Answer from the drawing. Dimensions are ordinates in mm from the lowest x, y and z of the part. Coordinates: 2 decimals unless noted, no trailing zeros. Loops run counter-clockwise (first coordinate to the right, second up) from the corner with the lowest first, then second, coordinate; pieces in that order, holes last. Notation, with made-up numbers: M 71,28.25 L 78,28.25 A16 cw 78,58.25 Z; hole C 70.5,30 d11. An arc over 180 degrees is marked long. Put each result on its own line as item: value.
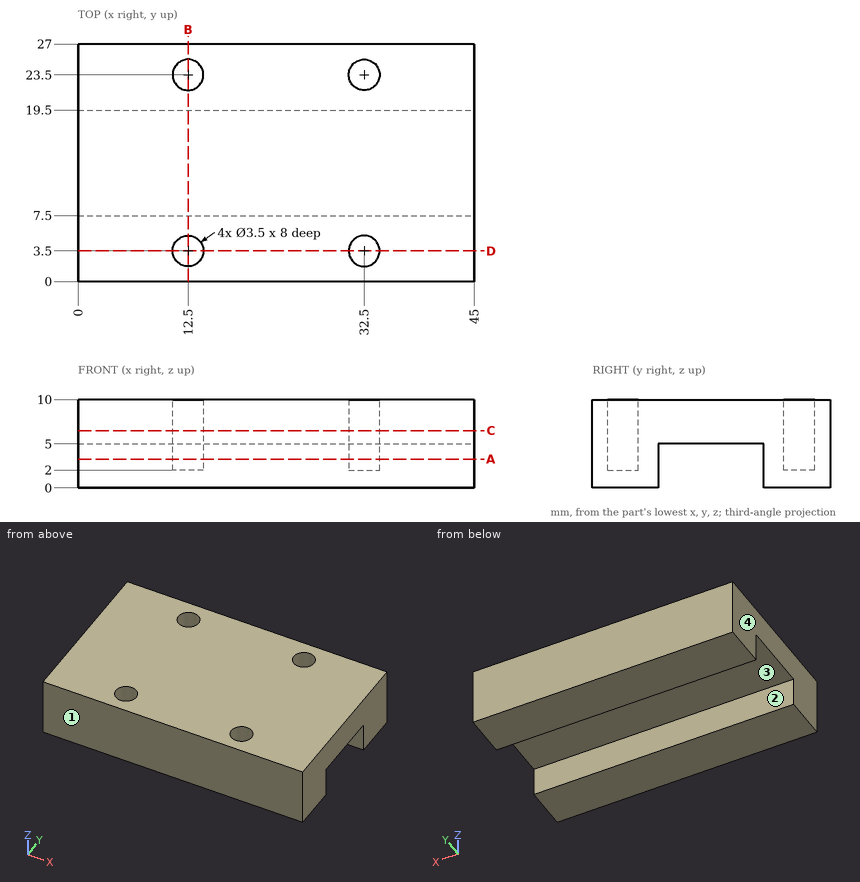
1) Determine the mould class of the marked faces 1, 2, 3 and 4 for opening direction Y: released by +Y, released by -Y, zero draft, split by the parting line, or undercut.
Answer list:
face 1: released by -Y
face 2: undercut
face 3: undercut
face 4: zero draft
2) Find section C-C, the plane z = 6.5. Write down the section's boundary in (x, y).
Answer list:
outline: M 0,0 L 45,0 L 45,27 L 0,27 Z; hole C 12.5,3.5 d3.5; hole C 12.5,23.5 d3.5; hole C 32.5,3.5 d3.5; hole C 32.5,23.5 d3.5
3) Given pin 1 Ø6 at (x, y) = (18.5, 12) entering from -Z; pin 2 Ø1 at (x, y) = (32, 4) entering from +Z, each flat-ended and moving along its own axis, determine where each tip first touches the part or whether it passes through.
Answer list:
pin 1: stops at z = 5
pin 2: stops at z = 2
4) Find section D-D, the plane y = 3.5. Write down the section's boundary in (x, z), plus the area to 3 significant figures.
Answer list:
outline: M 0,0 L 45,0 L 45,10 L 34.25,10 L 34.25,2 L 30.75,2 L 30.75,10 L 14.25,10 L 14.25,2 L 10.75,2 L 10.75,10 L 0,10 Z
area: 394 mm^2
5) Straight lines are drawn through the part: line 1 (Y direction, x = 32.5, z = 4); line 2 (X direction, y = 3.5, z = 6); line 3 (Y direction, x = 36.5, z = 1.25). For each, find the intervals that lie inside material, in ascending order. Write a range as [from, to].
Answer list:
line 1: y = [0, 1.75], [5.25, 7.5], [19.5, 21.75], [25.25, 27]
line 2: x = [0, 10.75], [14.25, 30.75], [34.25, 45]
line 3: y = [0, 7.5], [19.5, 27]
6) Find section B-B, the plane x = 12.5. Write down the section's boundary in (y, z), plus the area to 3 significant figures.
Answer list:
outline: M 0,0 L 7.5,0 L 7.5,5 L 19.5,5 L 19.5,0 L 27,0 L 27,10 L 25.25,10 L 25.25,2 L 21.75,2 L 21.75,10 L 5.25,10 L 5.25,2 L 1.75,2 L 1.75,10 L 0,10 Z
area: 154 mm^2
7) Find section A-A, the plane z = 3.25. Write down the section's boundary in (x, y).
Answer list:
outline: M 0,0 L 45,0 L 45,7.5 L 0,7.5 Z; M 0,19.5 L 45,19.5 L 45,27 L 0,27 Z; hole C 12.5,3.5 d3.5; hole C 12.5,23.5 d3.5; hole C 32.5,3.5 d3.5; hole C 32.5,23.5 d3.5
